from build123d import *

# Parameters (mm, degrees)
SKETCH1_R                                        = 36.5125
EXTRUDE1_DEPTH                                   = 9.525
SKETCH2_R                                        = 17.4625
SHAFT_THRU_HOLE_DEPTH                            = 53.507627422
CBORE_FOR_1_4_SOCKET_HEAD_CAP_SCREW1_D           = 6.7564
CBORE_FOR_1_4_SOCKET_HEAD_CAP_SCREW1_CBORE_D     = 11.1125
CBORE_FOR_1_4_SOCKET_HEAD_CAP_SCREW1_CBORE_DEPTH = 6.35


with BuildPart() as part:
    # Sketch1 → Extrude1 (new body)
    with BuildSketch(Plane.XY):
        with Locations(Location((0, 0, 0), (0, 0, 180))):
            Circle(SKETCH1_R)
    extrude(amount=EXTRUDE1_DEPTH)

    # Sketch2 → Shaft thru hole (cut, through all)
    with BuildSketch(Plane(origin=(0, 0, 9.525), x_dir=(-1, 0, 0), z_dir=(0, 0, 1))):
        with Locations(Location((0, 0, 0), (0, 0, 90))):
            Circle(SKETCH2_R)
    extrude(amount=-SHAFT_THRU_HOLE_DEPTH, mode=Mode.SUBTRACT)

    # CBORE for 1/4 Socket Head Cap Screw1 (through all)
    with Locations(Plane.XY.offset(9.525)):
        with Locations((0, 31.75), (-31.75, 0), (31.75, 0), (0, -31.75)):
            CounterBoreHole(CBORE_FOR_1_4_SOCKET_HEAD_CAP_SCREW1_D / 2, CBORE_FOR_1_4_SOCKET_HEAD_CAP_SCREW1_CBORE_D / 2, CBORE_FOR_1_4_SOCKET_HEAD_CAP_SCREW1_CBORE_DEPTH)


solid = part.part
Verification items for the finished model (mm, model axes). A direction names the side the tool comes from. Coordinates: 2 decimals unless noted, no trailing zeros. Order: outer loops, then holes, each group sorted by start corner. A loop starts at its lowest first (then second) coordinate and runs counter-clockwise, first axis right, second up. Notation, with made-up numbers: M -35.75,0.5 L -4.75,0.5 A25 cw -4.75,15.5 Z; hole C 23.25,25 d3. An arc over 180 degrees is marked long. One line per item, written item: value. Start each with the question number.
Item 1: Access from +Z, -Z, +X, -X, +Y, -Y to the whole of each face (thin tool, end or side, straight path). Record for faces 4 (the cylindrical face through (26.197, 0.199, 6.394)), 5 (the cylindrical face through (0.73, 28.45, 1.57)).
Item 2: Gauge pin test, flat ends, axial feed: pin 1 (3 mm diameter, centred on x = -2.5, y = -31.5, fed in from +Z) (3 decimals); pin 2 (1 mm diameter, centred on y = 26, z = 8.5, fed in from +X); pin 3 (5 mm diameter, centred on x = 3, z = 5.5, fed in from -Y). Record the tip position at first contact, or that the pin passes through.
Item 3: Mould release check, pull along Y, two halves, no side actions. Record for faces 1 (the cylindrical face through (28.629, -1.294, 1.565)), 2 (the flat face through (9, 16, 0)), 3 (the cylindrical face through (-34.826, -10.967, 4.696)): released by +Y, released by -Y, zero draft, split by the parting line, or undercut.
Item 4: Scan lines: probe 1 along X at (y, z) = (0, 8.25); probe 2 along X at (y, z) = (-16, 0.75); probe 3 along X at (y, z) = (-20.5, 7.5). Record each from-to range of solid material in increasing order.
Item 5: Sectioned sample at A-A (y = 0). Enter the section's corners in (x, z) (1 decimal).
Item 6: Sectioned sample at D-D (x = 16.5). Enter the section's corners in (y, z) (3 decimals).
Item 7: Sectioned sample at C-C (z = 2.25). Count the separate pieces of the cut face and the enclosed holes in it, then the cut area to 3 significant figures.
Conclusion:
1. face 4: +Z
1. face 5: +Z, -Z
2. pin 1: stops at z = 3.175
2. pin 2: stops at x = 26.13
2. pin 3: stops at y = -36.45
3. face 1: undercut
3. face 2: zero draft
3. face 3: split by the parting line
4. probe 1: x = -26.19 to -17.46, 17.46 to 26.19
4. probe 2: x = -32.82 to -7, 7 to 32.82
4. probe 3: x = -30.21 to 30.21
5. outline: M -36.5,0 L -35.1,0 L -35.1,3.2 L -36.5,3.2 Z; M -28.4,0 L -17.5,0 L -17.5,9.5 L -26.2,9.5 L -26.2,3.2 L -28.4,3.2 Z; M 17.5,0 L 28.4,0 L 28.4,3.2 L 26.2,3.2 L 26.2,9.5 L 17.5,9.5 Z; M 35.1,0 L 36.5,0 L 36.5,3.2 L 35.1,3.2 Z
6. outline: M -32.572,0 L -5.717,0 L -5.717,9.525 L -32.572,9.525 Z; M 5.717,0 L 32.572,0 L 32.572,9.525 L 5.717,9.525 Z
7. separate pieces: 1
7. enclosed holes: 5
7. area: 3,090 mm^2
